The model under review builds one solid part; all positions refer to its coordinate system, in mm. Face numbers are marked on the shaded views. A direction names the side the tool comes from. Coordinates: 2 decimals unless noted, no trailing zeros. Loops run counter-clockwise (first coordinate to the right, second up) from the corner with the lowest first, then second, coordinate; pieces in that order, holes last. Notation, with made-up numbers: M 4.25,-3.5 L 41.25,-3.5 A26 ccw 41.25,14.5 Z; hole C 72.5,75.5 d3. An arc over 180 degrees is marked long. Return JSON: item names as keys, results as strings.
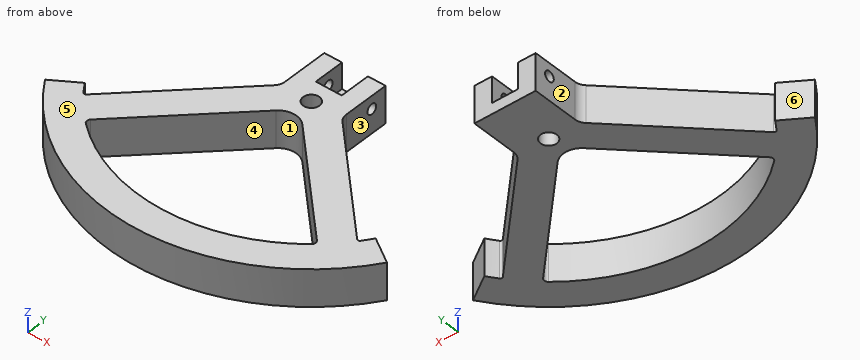
```python
from build123d import *

# Parameters (mm, degrees)
ESQUISSE1_R             = 4
BOSS_EXTRU_1_DEPTH      = 18
ESQUISSE2_W             = 12.7
ESQUISSE2_H             = 12.7
ENL_V_MAT_EXTRU_1_DEPTH = 15
ESQUISSE3_R             = 2.5
ENL_V_MAT_EXTRU_2_DEPTH = 30
CONG_1_R                = 1
CONG_2_R                = 6


with BuildPart() as part:
    # Esquisse1 → Boss.-Extru.1 (new body)
    with BuildSketch(Plane.XY):
        with BuildLine():
            Line((15, 25), (-15, 25))
            Line((-15, 25), (-15, 0))
            Line((-15, 0), (-67.134302209, -52.134302209))
            ThreePointArc((-67.134302209, -52.134302209), (-69.224071464, -49.325732939), (-71.196421393, -46.433496324))
            Line((-71.196421393, -46.433496324), (-83.760495756, -54.627642734))
            ThreePointArc((-83.760495756, -54.627642734), (0, -100), (83.760495756, -54.627642734))
            Line((83.760495756, -54.627642734), (71.196421393, -46.433496324))
            ThreePointArc((71.196421393, -46.433496324), (69.224071464, -49.325732939), (67.134302209, -52.134302209))
            Line((67.134302209, -52.134302209), (15, 0))
            Line((15, 0), (15, 25))
        make_face()
        Circle(ESQUISSE1_R, mode=Mode.SUBTRACT)
        with BuildLine():
            Line((-55.408885371, -61.622088806), (-6.464466094, -12.67766953))
            ThreePointArc((-6.464466094, -12.67766953), (0, -10), (6.464466094, -12.67766953))
            Line((6.464466094, -12.67766953), (55.408885371, -61.622088806))
            ThreePointArc((55.408885371, -61.622088806), (55.993185687, -63.113388543), (55.295748237, -64.555249414))
            ThreePointArc((55.295748237, -64.555249414), (0, -85), (-55.295748237, -64.555249414))
            ThreePointArc((-55.295748237, -64.555249414), (-55.993185687, -63.113388543), (-55.408885371, -61.622088806))
        make_face(mode=Mode.SUBTRACT)
    extrude(amount=BOSS_EXTRU_1_DEPTH)

    # Esquisse2 → Enlèv. mat.-Extru.1 (cut)
    with BuildSketch(Plane(origin=(0, 25, 0), x_dir=(1, 0, 0), z_dir=(0, 1, 0))):
        with Locations((0, -11.65)):
            Rectangle(ESQUISSE2_W, ESQUISSE2_H)
    extrude(amount=-ENL_V_MAT_EXTRU_1_DEPTH, mode=Mode.SUBTRACT)

    # Esquisse3 → Enlèv. mat.-Extru.2 (cut)
    with BuildSketch(Plane.ZY.offset(15)):
        with Locations((11.65, 17.125)):
            Circle(ESQUISSE3_R)
    extrude(amount=-ENL_V_MAT_EXTRU_2_DEPTH, mode=Mode.SUBTRACT)

    # Congé1
    cong_1_edges = [part.edges().sort_by_distance(p)[0] for p in [
        (67.134302209, -52.134302209, 9),
        (-67.134302209, -52.134302209, 9),
    ]]
    fillet(cong_1_edges, radius=CONG_1_R)

    # Congé2
    cong_2_edges = [part.edges().sort_by_distance(p)[0] for p in [
        (15, 0, 9),
        (-15, 0, 9),
    ]]
    fillet(cong_2_edges, radius=CONG_2_R)


solid = part.part
```
1. Add section D-D on z = 2.25. Give the boundary of the cut face in (x, y).
Check values:
{"outline": "M -83.76,-54.63 A100 ccw 83.76,-54.63 L 71.2,-46.43 A85 cw 67.83,-51.22 A1 cw 66.33,-51.33 L 16.76,-1.76 A6 cw 15,2.49 L 15,25 L -15,25 L -15,2.49 A6 cw -16.76,-1.76 L -66.33,-51.33 A1 cw -67.83,-51.22 A85 cw -71.2,-46.43 Z; hole M -55.41,-61.62 A2 ccw -55.3,-64.56 A85 ccw 55.3,-64.56 A2 ccw 55.41,-61.62 L 6.46,-12.68 A9.14 ccw -6.46,-12.68 Z; hole C 0,0 d8"}
2. Add section B-B on x = 0. Give the boundary of the cut face in (y, z).
Check values:
{"outline": "M -100,0 L -85,0 L -85,18 L -100,18 Z; M -10,0 L -4,0 L -4,18 L -10,18 Z; M 4,0 L 25,0 L 25,5.3 L 10,5.3 L 10,18 L 4,18 Z"}
3. Add section A-A on z = 11.65. State how many separate pieces and enclosed holes the cut face has, plus the area to 3 significant figures.
Check values:
{"separate pieces": "3", "enclosed holes": "2", "area": "5,610 mm²"}
4. Insertion check: pin 1 Ø4 at (y, z) = (17.5, 13) entering from +X; pin 2 Ø6 at (x, z) = (55.5, 7.5) entering from -Y; pin 3 Ø5.5 at (y, z) = (10.5, 8.5) entering from -X. Each pin has a flat end and moves straight along its axis. Give the tip position at first contact, or say it passes through.
Check values:
{"pin 1": "x = 15", "pin 2": "y = -85.11", "pin 3": "x = -15"}
5. To check wall thickness, follow line 1 (Y direction, x = -0.5, z = 4); line 2 (Y direction, x = 11.75, z = 11.65) (3 decimals); line 3 (Z direction, x = -6.5, y = 17). State the ranges of each line that lie inside material, in increasing order.
Check values:
{"line 1": "-100 to -85, -10.01 to -3.97, 3.97 to 25", "line 2": "-99.307 to -84.184, -17.963 to 14.625, 19.625 to 25", "line 3": "0 to 9.15, 14.15 to 18"}
6. Add section C-C on y = -83. Give the boundary of the cut face in (x, z), plus the area to 3 significant figures.
Check values:
{"outline": "M -55.78,0 L -18.33,0 L -18.33,18 L -55.78,18 Z; M 18.33,0 L 55.78,0 L 55.78,18 L 18.33,18 Z", "area": "1,350 mm²"}
7. Machinability: for the marked faces 1, 2 and 3, which of the approach directions +Z, -Z, +X, -X, +Y, -Y give a long, thin tool a straight path to every point of the face, cutting with its end or side? Answer none if there is none.
Check values:
{"face 1": "+Z, -Z", "face 2": "+Z, -Z, -X, +Y", "face 3": "+Z, -Z, +X, +Y"}
8. The part is to be moulded in two halves that separate along X. For the marked faces 4, 5 and 6, say which applies: released by +X, released by -X, zero draft, split by the parting line, or undercut.
Check values:
{"face 4": "undercut", "face 5": "zero draft", "face 6": "released by -X"}
